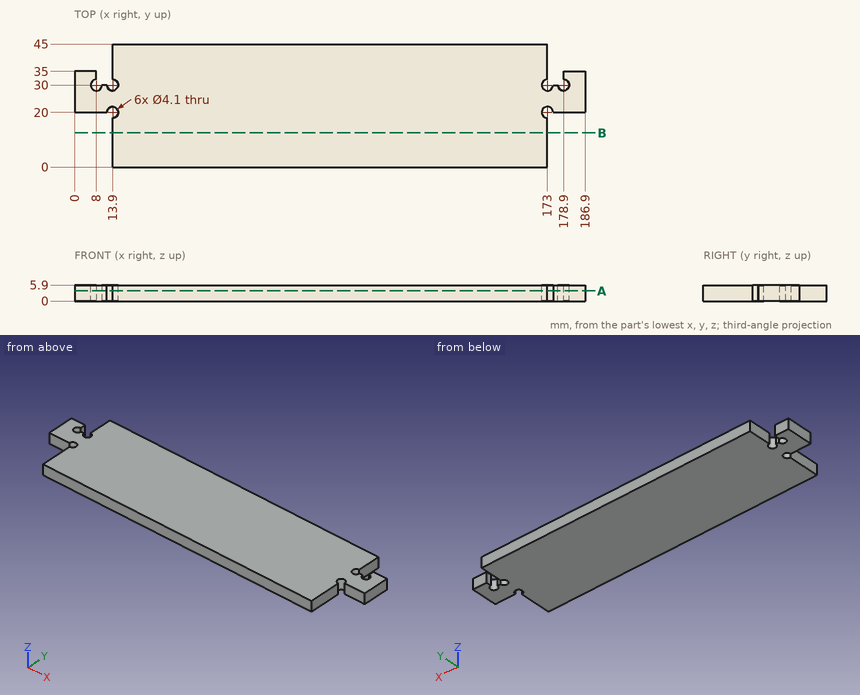
Could you check a few things on this drawing? It's one solid part, dimensions in mm from its lowest x, y, z. Round coordinates to 2 decimals unless told otherwise and drop trailing zeros. Write each loop counter-clockwise with the first axis right and the second up, starting at its lowest first coordinate (ties: lowest second). Pieces come first, ordered by that corner, then holes. Notation, with made-up numbers: (-6, -3) -> (0, -3) arc R24 ccw to (0, 26) -> close; hole circle Ø8 at (-6, -8). An arc over 180 degrees is marked (long way). One line per question, with ' | ' between items. Start each with the question number.
1) I'm going to push flat-ended pins straight in: P1, Ø3, axis at x = 182.5, z = 4, coming from the -Y side; P2, Ø2, axis at x = 176, z = 2, coming from the +Y side. Where does each tip first touch, or does it pass through?
2) Suppose I cut it at A-A on z = 3.8. Write out the boundary of the cut face in (x, y).
3) Suppose I cut it at B-B on y = 12.5. Write out the boundary of the cut face in (x, z), then the cut area to 3 significant figures.
4) I need wall thicknesses on line 1 (Y direction, x = 176, z = 2.35); line 2 (X direction, y = 12, z = 2.85). Which ranges of each line are inside material? Lowest first, please. Write a range as [from, to].
Return value:
1) P1: stops at y = 20 | P2: stops at y = 30
2) outline: (0, 20) -> (11.85, 20) arc R2.05 cw (long way) to (13.9, 17.95) -> (13.9, 0) -> (173, 0) -> (173, 17.95) arc R2.05 cw (long way) to (175.05, 20) -> (186.9, 20) -> (186.9, 35) -> (178.9, 35) -> (178.9, 32.05) arc R2.05 cw (long way) to (176.85, 30) -> (175.05, 30) arc R2.05 cw (long way) to (173, 32.05) -> (173, 45) -> (13.9, 45) -> (13.9, 32.05) arc R2.05 cw (long way) to (11.85, 30) -> (10.05, 30) arc R2.05 cw (long way) to (8, 32.05) -> (8, 35) -> (0, 35) -> close
3) outline: (13.9, 0) -> (173, 0) -> (173, 5.9) -> (13.9, 5.9) -> close | area: 939 mm2
4) line 1: y = [20, 30] | line 2: x = [13.9, 173]
